For this review, use the dimensioned drawing (mm, ordinates from the lowest corner) and the shaded views. Coordinates: 2 decimals unless noted, no trailing zeros. Order: outer loops, then holes, each group sorted by start corner. A loop starts at its lowest first (then second) coordinate and runs counter-clockwise, first axis right, second up. Notation, with made-up numbers: M -3,41 L 27,41 A22 ccw 27,59 Z; hole C 83,-31 d5. An arc over 180 degrees is marked long. Answer in a Markdown table with one row per item.
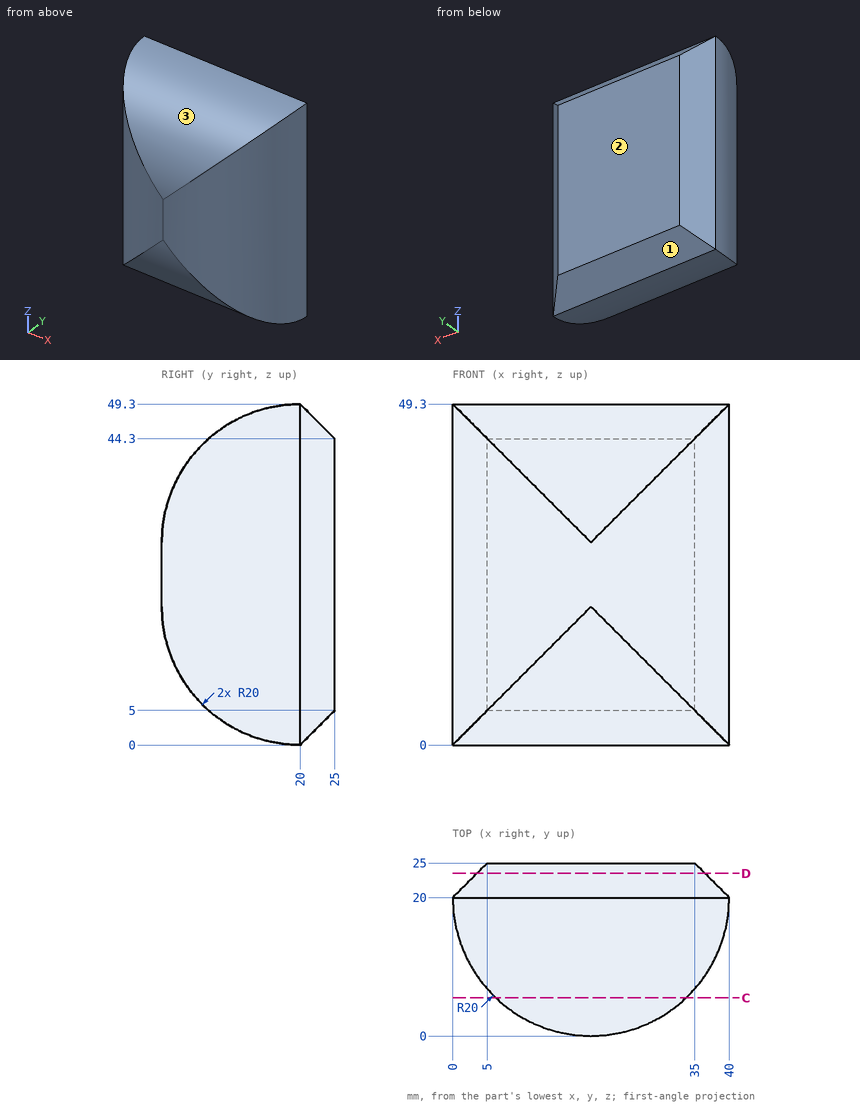
(1) Add section C-C, the plane y = 5.5. Give the boundary of the cut face in (x, z) (3 decimals).
Return value:
| item | result |
|---|---|
| outline | M 6.225,6.225 L 33.775,6.225 L 33.775,43.075 L 6.225,43.075 Z |
(2) Insertion check: pin 1 Ø4 at (y, z) = (14.5, 34.5) entering from +X; pin 2 Ø6 at (x, y) = (5, 12.5) entering from +Z; pin 3 Ø3 at (y, z) = (6.5, 11.5) entering from +X. Each pin has a flat end and moves straight along its axis. Give the tip position at first contact, or say it passes through.
Return value:
| item | result |
|---|---|
| pin 1 | stops at x = 39.69 |
| pin 2 | stops at z = 48.79 |
| pin 3 | stops at x = 36 |
(3) Add section D-D, the plane y = 23.5. Give the boundary of the cut face in (x, z), and give its area (3 significant figures).
Return value:
| item | result |
|---|---|
| outline | M 3.5,3.5 L 36.5,3.5 L 36.5,45.8 L 3.5,45.8 Z |
| area | 1,400 mm2 |
(4) Draft analysis for pull direction Z (two halves, no side actions). For the marked faces 1, 2 and 3, state which applies: pulls with the +Z half, pulls with the -Z half, needs draft (parallel to the pull), parting line crosses it, or undercut.
Return value:
| item | result |
|---|---|
| face 1 | pulls with the -Z half |
| face 2 | needs draft |
| face 3 | pulls with the +Z half |
(5) For line 1 along Z through (x, y) = (22.5, 22.75); line 2 along Y through (x, z) = (12.5, 30); line 3 along Y through (x, z) = (30, 35), list the stretches that pass through material, from the lowest coordinate up. Write a range as from..to.
Return value:
| item | result |
|---|---|
| line 1 | z = 2.75..46.55 |
| line 2 | y = 1.46..25 |
| line 3 | y = 2.68..25 |
